Autodesk Inventor part; units mm, degrees
ref_plane "YZ Plane" through (0, 0, 0) normal (1, 0, 0) x (0, 1, 0)
ref_plane "XZ Plane" through (0, 0, 0) normal (0, 1, 0) x (-1, 0, 0)
ref_plane "XY Plane" through (0, 0, 0) normal (0, 0, 1) x (1, 0, 0)
sketch "Sketch1" plane through (0, 0, 0) normal (1, 0, 0) x (0, 1, 0)
  line L0 (0, 0) -> (4.7625, 0)
  line L1 (4.7625, 0) -> (4.7625, 1.5875)
  line L2 (4.7625, 1.5875) -> (7.9375, 1.5875)
  line L3 (7.9375, 1.5875) -> (7.9375, 0)
  line L4 (7.9375, 0) -> (6.35, 0)
  line L5 (6.35, 0) -> (6.35, -6.35)
  line L6 (6.35, -6.35) -> (4.7625, -6.35)
  line L7 (4.7625, -6.35) -> (4.7625, 0)
  line L8 (0, 0) -> (0, -7.0209)
  dimension "d0" = 9.525
  dimension "d1" = 12.7
  dimension "d2" = 15.875
  dimension "d3" = 1.5875
  dimension "d4" = 6.35
revolve "Revolution1" add sketch "Sketch1" angle 360 about axis through (0, 0, 0) along (0, 0, -1)
sketch "Sketch2" plane through (0, 0, -6.35) normal (0, 0, -1) x (-1, 0, 0)
  circle A0 centre (0, 0) radius 6.35
  line L0 (-7.3323, 0) -> (-3.6662, 6.35)
  line L1 (-3.6662, 6.35) -> (3.6662, 6.35)
  line L2 (3.6662, 6.35) -> (7.3323, 0)
  line L3 (7.3323, 0) -> (3.6662, -6.35)
  line L4 (3.6662, -6.35) -> (-3.6662, -6.35)
  line L5 (-3.6662, -6.35) -> (-7.3323, 0)
  point P0 (-5.4993, -3.175)
  point P1 (0, -6.35)
  point P2 (-5.4993, 3.175)
  point P3 (5.4993, -3.175)
  point P4 (5.4993, 3.175)
  point P5 (0, 6.35)
extrude "Extrusion1" add sketch "Sketch2" against normal up to surface (6.35 mm away) contours A0 L2 L3 | A0 L1 L2 | L3 L4 A0 | A0 L0 L1 | L4 L5 A0 | A0 L5 L0
chamfer "Chamfer1" distance 0.127 angle 45 2 edges at (0, -7.9375, 1.5875) (0, -4.7625, 1.5875)
properties part number "WCP 500 Hex Bushing" material "Brass, Soft Yellow"
The listing builds one solid part. Answer for the finished solid, in the listing's coordinates (mm). A direction names the side the tool comes from. Coordinates: 2 decimals unless noted, no trailing zeros. Write each loop counter-clockwise with the first axis right and the second up, starting at its lowest first coordinate (ties: lowest second). Pieces come first, ordered by that corner, then holes. Notation, with made-up numbers: M 83,-35.75 L 89,-35.75 A4 cw 89,-28.75 Z; hole C 35,86 d10. An arc over 180 degrees is marked long. Write each question's results on one line, items separated by ' | '.
Item 1: For a pull along Y with two mould halves and no side action, classify faces 1 (the face through (0, -6.35, -3)), 2 (the face through (2.9, -3.78, -2.39)), 3 (the face through (-5.474, 3.219, -3.219)) as released by +Y, released by -Y, zero draft, split by the parting line, or undercut.
Answer below:
face 1: released by -Y | face 2: undercut | face 3: released by +Y
Item 2: The part is cut by section A-A on x = 0. Determine the outline of the cut face in (y, z), and give its area (3 significant figures).
Answer below:
outline: M -7.94,0 L -6.35,0 L -6.35,-6.35 L -4.76,-6.35 L -4.76,1.46 L -4.89,1.59 L -7.81,1.59 L -7.94,1.46 Z; M 4.76,-6.35 L 6.35,-6.35 L 6.35,0 L 7.94,0 L 7.94,1.46 L 7.81,1.59 L 4.89,1.59 L 4.76,1.46 Z | area: 30.2 mm2
Item 3: Consider probe 1 along X at (y, z) = (-3.75, -2); probe 2 along X at (y, z) = (0, 0.25); probe 3 along Y at (x, z) = (4, -3.25). Determine where each line is inside the solid, lowest interval first. Write a range as [from, to].
Answer below:
probe 1: [-5.17, -2.94], [2.94, 5.17] | probe 2: [-7.94, -4.76], [4.76, 7.94] | probe 3: [-5.77, -2.58], [2.58, 5.77]
Item 4: Given P1, Ø1, axis at y = 3.5, z = 0.5, coming from the -X side; P2, Ø8, axis at x = 0, y = 1.5, coming from the -Z side; P3, Ø4, axis at x = -4.5, z = -4.5, coming from the +Y side; P4, Ø8.5, axis at x = 0, y = 0, coming from the -Z side, each flat-ended and moving along its own axis, determine where each tip first touches the part or whether it passes through.
Answer below:
P1: x = -7.35 | P2: z = -6.35 | P3: y = 6.35 | P4: through
Item 5: Which of the six approach directions +Z, -Z, +X, -X, +Y, -Y give full straight-line access (tool end or side, diameter ignored) to faces 4 (the face through (6, 3, 0)), 5 (the face through (5.474, -3.219, -3.219)), 6 (the face through (5.525, 3.131, -3.219))?
Answer below:
face 4: -Z | face 5: -Z, +X, -Y | face 6: -Z, +X, +Y
